The listing builds one solid part. Answer for the finished solid, in the listing's coordinates (mm). Face numbers are marked on the shaded views. A direction names the side the tool comes from. Coordinates: 2 decimals unless noted, no trailing zeros. Order: outer loops, then holes, each group sorted by start corner. A loop starts at its lowest first (then second) coordinate and runs counter-clockwise, first axis right, second up. Notation, with made-up numbers: (79, -36.75) - (83, -36.75) arc R16 ccw to (83, -6.75) - close; hole circle Ø9 at (56, -20). An arc over 180 degrees is marked (long way). Use a Markdown table: item, result. Add a question column.
Item 1: For the marked faces 5 and 6, determine the directions among +Z, -Z, +X, -X, +Y, -Y from which every point of the face is accessible in a straight line to the end or side of a thin tool.
Item 2: The mould has two halves that part along X. Classify the marked faces 1, 2, 3 and 4: released by +X, released by -X, zero draft, split by the parting line, or undercut.
Item 3: The part is cut by section A-A, the plane z = 31.5. Give the vertices of the cut face in (x, y), then the cut area to 3 significant figures.
Item 4: The part is cut by section B-B, the plane y = -15.5. Give the vertices of the cut face in (x, z).
Item 5: Flat-ended cylindrical pins translate along their axes: P1, Ø5, axis at x = -26.99, z = 8, coming from the +Y side; P2, Ø3, axis at x = -25.5, y = 16.5, coming from the +Z side; P3, Ø8, axis at y = 10, z = 23, coming from the -X side; P4, Ø13, axis at x = 20, y = -5, coming from the +Z side. Find the tip coordinate at first contact, or state that the pin passes through.
Item 6: The part is cut by section C-C, the plane z = 44. Give the vertices of the cut face in (x, y), then the cut area to 3 significant figures.
Item 7: The part is cut by section D-D, the plane x = 11. Give the vertices of the cut face in (y, z), then the cut area to 3 significant figures.
Item 8: Find the intervals of material crossed by line 1 along Z through (x, y) = (39.5, 8.5); line 2 along X through (y, z) = (-14, 14.5); line 3 along Z through (x, y) = (4, 5), in increasing order.
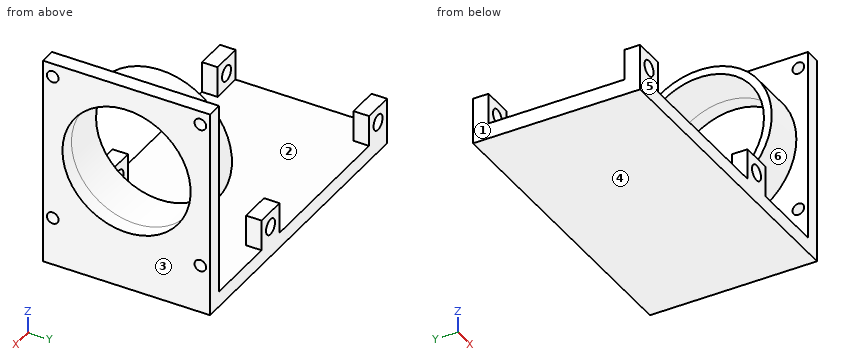
from build123d import *

# Parameters (mm, degrees)
F0_W      = 79
F0_H      = 43
F1_DEPTH  = 4
F2_W      = 4
F2_H      = 43
F3_DEPTH  = 50
F4_W      = 8
F4_H      = 4
F5_DEPTH  = 8
F6_W      = 8
F6_H      = 4
F7_DEPTH  = 8
F8_W      = 8
F8_H      = 4
F9_DEPTH  = 8
F10_W     = 8
F10_H     = 4
F11_DEPTH = 8
F13_D     = 4
F13_DEPTH = 4.001
F15_D     = 4
F15_DEPTH = 4.001
F17_D     = 4
F19_D     = 4
F21_D     = 33
F22_R     = 18.5
F22_R_2   = 16.5
F23_DEPTH = 11
F25_D     = 3
F27_D     = 3
F29_D     = 3
F29_DEPTH = 12
F29_TIP   = 0.9012909285
F31_D     = 3
F31_DEPTH = 12
F31_TIP   = 0.9012909285


with BuildPart() as f1:
    # F0 (on Top) → F1 (new body)
    with BuildSketch(Plane.XY):
        with Locations((8.5094775558, -3.8157299012)):
            Rectangle(F0_W, F0_H)
    extrude(amount=F1_DEPTH)

    # F2 (on face) → F3 (join)
    with BuildSketch(Plane.XY.offset(4)):
        with Locations((46.0094775558, -3.8157299012)):
            Rectangle(F2_W, F2_H)
    extrude(amount=F3_DEPTH)

    # F4 (on face) → F5 (join)
    with BuildSketch(Plane.XY.offset(4)):
        with Locations((-26.9905224442, -23.3157299012)):
            Rectangle(F4_W, F4_H)
    extrude(amount=F5_DEPTH)

    # F6 (on face) → F7 (join)
    with BuildSketch(Plane.XY.offset(4)):
        with Locations((-26.9905224442, 15.6842700988)):
            Rectangle(F6_W, F6_H)
    extrude(amount=F7_DEPTH)

    # F8 (on face) → F9 (join)
    with BuildSketch(Plane.XY.offset(4)):
        with Locations((21.0094775558, 15.6842700988)):
            Rectangle(F8_W, F8_H)
    extrude(amount=F9_DEPTH)

    # F10 (on face) → F11 (join)
    with BuildSketch(Plane.XY.offset(4)):
        with Locations((21.0094775558, -23.3157299012)):
            Rectangle(F10_W, F10_H)
    extrude(amount=F11_DEPTH)

    # F13 (through all, one way)
    with BuildSketch(Plane.XZ.offset(-13.6842700988)):
        with Locations((-26.9905224442, 8)):
            Circle(F13_D / 2)
    extrude(amount=-F13_DEPTH, mode=Mode.SUBTRACT)

    # F15 (through all, one way)
    with BuildSketch(Plane.XZ.offset(-13.6842700988)):
        with Locations((21.0094775558, 8)):
            Circle(F15_D / 2)
    extrude(amount=-F15_DEPTH, mode=Mode.SUBTRACT)

    # F17 (through all)
    with Locations(Plane(origin=(0, -21.3157299012, 0), x_dir=(-1, 0, 0), z_dir=(0, 1, 0))):
        with Locations((26.9905224442, 8)):
            Hole(F17_D / 2)

    # F19 (through all)
    with Locations(Plane(origin=(0, -21.3157299012, 0), x_dir=(-1, 0, 0), z_dir=(0, 1, 0))):
        with Locations((-21.0094775558, 8)):
            Hole(F19_D / 2)

    # F21 (through all)
    with Locations(Plane.YZ.offset(48.0094775558)):
        with Locations((-3.8157299012, 31.5)):
            Hole(F21_D / 2)

    # F22 (on face) → F23 (join)
    with BuildSketch(Plane(origin=(44.0094775558, 0, 0), x_dir=(0, -1, 0), z_dir=(-1, 0, 0))):
        with Locations((3.8157299012, 31.5)):
            Circle(F22_R)
        with Locations((3.8157299012, 31.5)):
            Circle(F22_R_2, mode=Mode.SUBTRACT)
    extrude(amount=F23_DEPTH)

    # F25 (through all)
    with Locations(Plane.YZ.offset(48.0094775558)):
        with Locations((-22.8157299012, 50.5)):
            Hole(F25_D / 2)

    # F27 (through all)
    with Locations(Plane.YZ.offset(48.0094775558)):
        with Locations((15.1842700988, 50.5)):
            Hole(F27_D / 2)

    # F29
    with Locations(Plane.YZ.offset(48.0094775558)):
        with Locations((-22.8157299012, 12.5)):
            Hole(F29_D / 2, depth=F29_DEPTH)
            with Locations((0, 0, -(F29_DEPTH + F29_TIP / 2))):  # 118° drill point
                Cone(0, F29_D / 2, F29_TIP, mode=Mode.SUBTRACT)

    # F31
    with Locations(Plane.YZ.offset(48.0094775558)):
        with Locations((15.1842700988, 12.5)):
            Hole(F31_D / 2, depth=F31_DEPTH)
            with Locations((0, 0, -(F31_DEPTH + F31_TIP / 2))):  # 118° drill point
                Cone(0, F31_D / 2, F31_TIP, mode=Mode.SUBTRACT)


solid = f1.part
Solution:
| question | item | result |
|---|---|---|
| 1 | face 5 | +Z, -Z, +X, -X, -Y |
| 1 | face 6 | -X |
| 2 | face 1 | released by -X |
| 2 | face 2 | undercut |
| 2 | face 3 | released by +X |
| 2 | face 4 | zero draft |
| 3 | outline | (33.01, -22.32) - (44.01, -22.32) - (44.01, -25.32) - (48.01, -25.32) - (48.01, -20.32) - (33.01, -20.32) - close; (33.01, 12.68) - (48.01, 12.68) - (48.01, 17.68) - (44.01, 17.68) - (44.01, 14.68) - (33.01, 14.68) - close |
| 3 | area | 84.0 mm2 |
| 4 | outline | (-30.99, 0) - (48.01, 0) - (48.01, 19.85) - (33.01, 19.85) - (33.01, 17.16) - (44.01, 17.16) - (44.01, 4) - (-30.99, 4) - close; (33.01, 43.15) - (48.01, 43.15) - (48.01, 54) - (44.01, 54) - (44.01, 45.84) - (33.01, 45.84) - close |
| 5 | P1 | stops at y = 17.68 |
| 5 | P2 | stops at z = 12 |
| 5 | P3 | stops at x = 33.01 |
| 5 | P4 | stops at z = 4 |
| 6 | outline | (33.01, -17.45) - (44.01, -17.45) - (44.01, -25.32) - (48.01, -25.32) - (48.01, -14.59) - (33.01, -14.59) - close; (33.01, 6.95) - (48.01, 6.95) - (48.01, 17.68) - (44.01, 17.68) - (44.01, 9.82) - (33.01, 9.82) - close |
| 6 | area | 149 mm2 |
| 7 | outline | (-25.32, 0) - (17.68, 0) - (17.68, 4) - (-25.32, 4) - close |
| 7 | area | 172 mm2 |
| 8 | line 1 | z = 0 to 4, 17.7 to 20.52, 42.48 to 45.3 |
| 8 | line 2 | x = 44.01 to 48.01 |
| 8 | line 3 | z = 0 to 4 |
